```python
from build123d import *

# Parameters (mm, degrees)
SKETCH_1_R      = 1.65
EXTRUDE_1_DEPTH = 3
EXTRUDE_START   = -3
EXTRUDE_2_DEPTH = 3


with BuildPart() as part:
    # 草图1 → 凸台-拉伸1 (new body)
    with BuildSketch(Plane.XY):
        with BuildLine():
            Line((4, 10), (4, -10))
            ThreePointArc((4, -10), (0, -14), (-4, -10))
            Line((-4, -10), (-4, 10))
            ThreePointArc((-4, 10), (0, 14), (4, 10))
        make_face()
        with Locations((0, 10)):
            Circle(SKETCH_1_R, mode=Mode.SUBTRACT)
        with Locations((0, -10)):
            Circle(SKETCH_1_R, mode=Mode.SUBTRACT)
    extrude(amount=EXTRUDE_1_DEPTH)

    # 草图2 → 凸台-拉伸2 (add)
    with BuildSketch(Plane.XY.offset(3).offset(EXTRUDE_START)):
        with BuildLine():
            Line((-4, 10), (-4, 25))
            Line((-4, 25), (4, 25))
            Line((4, 25), (4, 10))
            ThreePointArc((4, 10), (0, 14), (-4, 10))
        make_face()
    extrude(amount=EXTRUDE_2_DEPTH)


solid = part.part
```
Geometry: final body of the model. Coordinates: model frame, mm. Round coordinates to 2 decimals unless told otherwise and drop trailing zeros. Loops run counter-clockwise (first coordinate to the right, second up) from the corner with the lowest first, then second, coordinate; pieces in that order, holes last.
Item 1: Section D-D, the plane x = 3. Output: boundary loops of the cut face in (y, z), plus the area to 3 significant figures.
Checked values:
outline: (-12.65, 0) - (25, 0) - (25, 3) - (-12.65, 3) - close
area: 113 mm2
Item 2: Line query: L1, parallel to Y at x = 0, z = 2.2; L2, parallel to X at y = -9, z = 2.1; L3, parallel to Y at x = -3, z = 0.25. Output: solid intervals per line, ascending.
Checked values:
L1: y = -14 to -11.65, -8.35 to 8.35, 11.65 to 25
L2: x = -4 to -1.31, 1.31 to 4
L3: y = -12.65 to 25
Item 3: Section C-C, the plane z = 1.3. Output: boundary loops of the cut face in (x, y).
Checked values:
outline: (-4, -10) arc R4 ccw to (4, -10) - (4, 25) - (-4, 25) - close; hole circle Ø3.3 at (0, -10); hole circle Ø3.3 at (0, 10)
Item 4: Section A-A, the plane y = 10. Output: boundary loops of the cut face in (x, z).
Checked values:
outline: (-4, 0) - (-1.65, 0) - (-1.65, 3) - (-4, 3) - close; (1.65, 0) - (4, 0) - (4, 3) - (1.65, 3) - close
Item 5: Mould query, pull axis X, two halves, no side actions, for faces 1 (the flat face through (4, 8, 1)), 2 (the flat face through (0, 6, 3)), 3 (the cylindrical face through (-0.4, 8.4, 1.5)). Classes: released by +X, released by -X, zero draft, split by the parting line, or undercut.
Checked values:
face 1: released by +X
face 2: zero draft
face 3: undercut
Item 6: Section B-B, the plane x = 0. Output: boundary loops of the cut face in (y, z).
Checked values:
outline: (-14, 0) - (-11.65, 0) - (-11.65, 3) - (-14, 3) - close; (-8.35, 0) - (8.35, 0) - (8.35, 3) - (-8.35, 3) - close; (11.65, 0) - (25, 0) - (25, 3) - (11.65, 3) - close
